from build123d import *

# Parameters (mm, degrees)
BOSS_EXTRUDE1_DEPTH          = 3.175
F_3_8_0_375_DIAMETER_HOLE1_D = 9.525


with BuildPart() as part:
    # Sketch1 → Boss-Extrude1 (new body)
    with BuildSketch(Plane(origin=(0, 0, 0), x_dir=(1, 0, 0), z_dir=(0, 1, 0))):
        with BuildLine():
            Line((3.175, 0), (47.625, 0))
            ThreePointArc((47.625, 0), (49.87006403, 0.92993597), (50.8, 3.175))
            Line((50.8, 3.175), (50.8, 34.925))
            ThreePointArc((50.8, 34.925), (49.87006403, 37.17006403), (47.625, 38.1))
            Line((47.625, 38.1), (3.175, 38.1))
            ThreePointArc((3.175, 38.1), (0.92993597, 37.17006403), (0, 34.925))
            Line((0, 34.925), (0, 3.175))
            ThreePointArc((0, 3.175), (0.92993597, 0.92993597), (3.175, 0))
        make_face()
    extrude(amount=BOSS_EXTRUDE1_DEPTH)

    # 3/8 (0.375) Diameter Hole1 (through all)
    with Locations(Plane(origin=(0, 3.175, 0), x_dir=(1, 0, 0), z_dir=(0, 1, 0))):
        with Locations((19.05, 19.05)):
            Hole(F_3_8_0_375_DIAMETER_HOLE1_D / 2)


solid = part.part
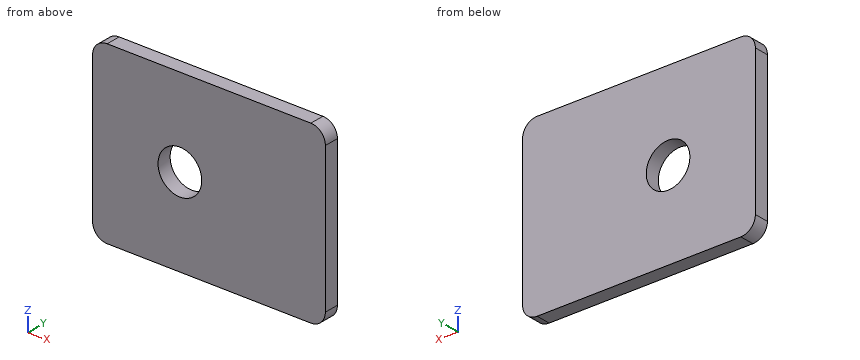
Design review of the part built by this model. Coordinates are the model's own, in mm. Give positions to 0.01 mm unless a question says otherwise; leave off trailing zeros. Write each loop counter-clockwise with the first axis right and the second up, starting at its lowest first coordinate (ties: lowest second). Pieces come first, ordered by that corner, then holes. Notation, with made-up numbers: M 83,36.5 L 135,36.5 A6 ccw 135,41.5 Z; hole C -14,32.5 d9. An arc over 180 degrees is marked long. Answer as a JSON object with one key per item and string values. Group by question number.
1) We need section C-C (z = -19.05). Give the boundary of the cut face in (x, y) (1 decimal).
2) Clearance check with a flat-ended pin moving along its axis: pin 1 Ø4 at (x, z) = (27.5, -20.5) entering from -Y. State where the tip first meets the part, or that it passes through.
3) We need section A-A (x = 19.05). Give the boundary of the cut face in (y, z) (1 decimal).
4) For line 1 along X through (y, z) = (1.2, -19.05); line 2 along Z through (x, y) = (19.05, 2.05); line 3 along X through (y, z) = (2.6, -35), list the stretches that pass through material, from the lowest coordinate up.
Answer key:
{
 "1": {"outline": "M 0,0 L 14.3,0 L 14.3,3.2 L 0,3.2 Z; M 23.8,0 L 50.8,0 L 50.8,3.2 L 23.8,3.2 Z"},
 "2": {"pin 1": "stops at y = 0"},
 "3": {"outline": "M 0,-38.1 L 3.2,-38.1 L 3.2,-23.8 L 0,-23.8 Z; M 0,-14.3 L 3.2,-14.3 L 3.2,0 L 0,0 Z"},
 "4": {"line 1": "x = 0 to 14.29, 23.81 to 50.8", "line 2": "z = -38.1 to -23.81, -14.29 to 0", "line 3": "x = 0 to 50.8"}
}
